Geometry: final body of the model. Coordinates: model frame, mm. A direction names the side the tool comes from. Coordinates: 2 decimals unless noted, no trailing zeros. Write each loop counter-clockwise with the first axis right and the second up, starting at its lowest first coordinate (ties: lowest second). Pieces come first, ordered by that corner, then holes. Notation, with made-up numbers: (86, -23) -> (140, -23) arc R20 cw to (140, -12) -> close; hole circle Ø6 at (-11.75, 57.25). An arc over 180 degrees is marked (long way). Answer as a JSON object with one key per item and string values. Group by question number.
```python
from build123d import *

# Parameters (mm, degrees)
SKETCH030_R     = 10
PAD016_DEPTH    = 2
SKETCH031_R     = 5.5
POCKET011_DEPTH = 2.001
SKETCH032_W     = 2.6
SKETCH032_H     = 16
POCKET012_DEPTH = 2.001
SKETCH033_W     = 16
SKETCH033_H     = 6
POCKET013_DEPTH = 2.001


with BuildPart() as part:
    # Sketch030 → Pad016 (new body)
    with BuildSketch(Plane.XY):
        Circle(SKETCH030_R)
    extrude(amount=PAD016_DEPTH)

    # Sketch031 → Pocket011 (cut, through all)
    with BuildSketch(Plane.XY):
        Circle(SKETCH031_R)
    extrude(amount=POCKET011_DEPTH, mode=Mode.SUBTRACT)

    # Sketch032 → Pocket012 (cut, through all)
    with BuildSketch(Plane.XY):
        Rectangle(SKETCH032_W, SKETCH032_H)
    extrude(amount=POCKET012_DEPTH, mode=Mode.SUBTRACT)

    # Sketch033 → Pocket013 (cut, through all)
    with BuildSketch(Plane.XY):
        Rectangle(SKETCH033_W, SKETCH033_H)
    extrude(amount=POCKET013_DEPTH, mode=Mode.SUBTRACT)


solid = part.part
```
Item 1: Ray query, L1, parallel to Y at x = 0, z = 1.3; L2, parallel to X at y = 6, z = 1.3; L3, parallel to X at y = -3.5, z = 0.4. Return the intervals inside material, ascending. Write a range as [from, to].
Item 2: Section C-C on x = 6. Output: boundary loops of the cut face in (y, z), then the cut area to 3 significant figures.
Item 3: Set-up query: faces 1 (the cylindrical face through (3.155, -4.505, 0.986)), 2 (the flat face through (4, -4, 0)). Return all of +Z, -Z, +X, -X, +Y, -Y with unobstructed straight access to the full face (end or side cutting, diameter ignored); none if empty.
Item 4: Section B-B on y = 0. Output: boundary loops of the cut face in (x, z), then the cut area to 3 significant figures.
Item 5: Section A-A on z = 0.7. Output: boundary loops of the cut face in (x, y).
Item 6: Contact query for flat-ended pins moving along their axis: pin 1 (0.6 mm diameter, centred on y = -1.5, z = 1, fed in from +X); pin 2 (0.6 mm diameter, centred on x = -6.5, z = 1, fed in from -Y); pin 3 (0.6 mm diameter, centred on y = 6.5, z = 1, fed in from -X). Output: stop coordinate, or through.
Answer sheet:
{
 "1": {"L1": "y = [-10, -8], [8, 10]", "L2": "x = [-8, -1.3], [1.3, 8]", "L3": "x = [-9.37, -4.24], [4.24, 9.37]"},
 "2": {"outline": "(-8, 0) -> (-3, 0) -> (-3, 2) -> (-8, 2) -> close; (3, 0) -> (8, 0) -> (8, 2) -> (3, 2) -> close", "area": "20.0 mm^2"},
 "3": {"face 1": "+Z, -Z", "face 2": "-Z, +X, -X, +Y, -Y"},
 "4": {"outline": "(-10, 0) -> (-8, 0) -> (-8, 2) -> (-10, 2) -> close; (8, 0) -> (10, 0) -> (10, 2) -> (8, 2) -> close", "area": "8.00 mm^2"},
 "5": {"outline": "circle Ø20 at (0, 0); hole (-8, -3) -> (-4.61, -3) arc R5.5 ccw to (-1.3, -5.34) -> (-1.3, -8) -> (1.3, -8) -> (1.3, -5.34) arc R5.5 ccw to (4.61, -3) -> (8, -3) -> (8, 3) -> (4.61, 3) arc R5.5 ccw to (1.3, 5.34) -> (1.3, 8) -> (-1.3, 8) -> (-1.3, 5.34) arc R5.5 ccw to (-4.61, 3) -> (-8, 3) -> close"},
 "6": {"pin 1": "stops at x = 9.93", "pin 2": "stops at y = -7.85", "pin 3": "stops at x = -7.85"}
}
